```python
from build123d import *

# Parameters (mm, degrees)
SKETCH1_R               = 16
BOSS_EXTRUDE1_DEPTH     = 146
SKETCH2_W               = 150.836885197
SKETCH2_H               = 19.135619971
CUT_EXTRUDE2_DEPTH      = 17
CUT_EXTRUDE2_DEPTH_BACK = 17
SKETCH3_R               = 4
CUT_EXTRUDE3_DEPTH      = 15.463502114
CUT_EXTRUDE3_DEPTH_BACK = 15.463502114
SKETCH5_W               = 20
SKETCH5_H               = 24.196648242
CUT_EXTRUDE4_DEPTH      = 17.0000001
CUT_EXTRUDE4_DEPTH_BACK = 17.0000001
SKETCH6_R               = 4
CUT_EXTRUDE5_DEPTH      = 29


with BuildPart() as part:
    # Sketch1 → Boss-Extrude1 (new body)
    with BuildSketch(Plane.XY):
        Circle(SKETCH1_R)
    extrude(amount=BOSS_EXTRUDE1_DEPTH)

    # Sketch2 → Cut-Extrude2 (cut, two sides)
    with BuildSketch(Plane(origin=(0, 0, 0), x_dir=(0, 0, -1), z_dir=(1, 0, 0))) as cut_extrude2_sk:
        with BuildLine():
            Line((-116, -5), (-116, 5))
            ThreePointArc((-116, 5), (-116.878679656, 7.121320344), (-119, 8))
            Line((-119, 8), (-146, 8))
            Line((-146, 8), (-146, -8))
            Line((-146, -8), (-119, -8))
            ThreePointArc((-119, -8), (-116.878679656, -7.121320344), (-116, -5))
        make_face()
        with Locations((-70.581557402, -24.031312)):
            Rectangle(SKETCH2_W, SKETCH2_H)
        with Locations((-70.581557402, 24.031312)):
            Rectangle(SKETCH2_W, SKETCH2_H)
    extrude(amount=CUT_EXTRUDE2_DEPTH, mode=Mode.SUBTRACT)
    extrude(cut_extrude2_sk.sketch, amount=-CUT_EXTRUDE2_DEPTH_BACK, mode=Mode.SUBTRACT)

    # Sketch3 → Cut-Extrude3 (cut, two sides)
    with BuildSketch(Plane(origin=(0, 0, 0), x_dir=(1, 0, 0), z_dir=(0, 1, 0))) as cut_extrude3_sk:
        with Locations((0, -136)):
            Circle(SKETCH3_R)
    extrude(amount=CUT_EXTRUDE3_DEPTH, mode=Mode.SUBTRACT)
    extrude(cut_extrude3_sk.sketch, amount=-CUT_EXTRUDE3_DEPTH_BACK, mode=Mode.SUBTRACT)

    # Sketch4 → Cut-Revolve3 (revolve, cut)
    with BuildSketch(Plane(origin=(0, 0, 0), x_dir=(0, 0, -1), z_dir=(1, 0, 0))):
        with BuildLine():
            Line((0, 7), (-80, 7))
            ThreePointArc((-80, 7), (-86.772424654, 8.019684618), (-92.944350416, 10.988324842))
            Line((-92.944350416, 10.988324842), (-118.219798108, 28.197447612))
            Line((-118.219798108, 28.197447612), (0, 28.197447612))
            Line((0, 28.197447612), (0, 7))
        make_face()
    revolve(axis=Axis((0, 0, 0), (0, 0, 1)), mode=Mode.SUBTRACT)

    # Sketch5 → Cut-Extrude4 (cut, two sides)
    with BuildSketch(Plane(origin=(0, 0, 0), x_dir=(0, 0, -1), z_dir=(1, 0, 0))) as cut_extrude4_sk:
        with Locations((-10, 0)):
            Rectangle(SKETCH5_W, SKETCH5_H)
    extrude(amount=CUT_EXTRUDE4_DEPTH, mode=Mode.SUBTRACT)
    extrude(cut_extrude4_sk.sketch, amount=-CUT_EXTRUDE4_DEPTH_BACK, mode=Mode.SUBTRACT)

    # Sketch6 → Cut-Extrude5 (cut)
    with BuildSketch(Plane(origin=(0, 0, 20), x_dir=(-1, 0, 0), z_dir=(0, 0, -1))):
        Circle(SKETCH6_R)
    extrude(amount=-CUT_EXTRUDE5_DEPTH, mode=Mode.SUBTRACT)


solid = part.part
```
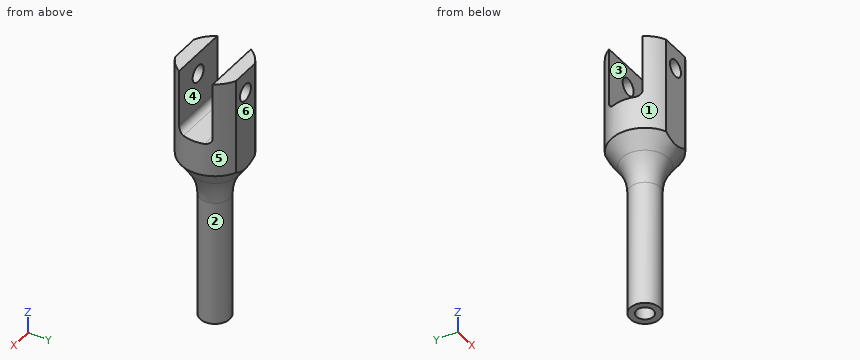
Here's how the part is built. I have some questions about the finished solid (model axes, mm). Face numbers are marked on the shaded views. A direction names the side the tool comes from. Give positions to 0.01 mm unless a question says otherwise; leave off trailing zeros. Loops run counter-clockwise (first coordinate to the right, second up) from the corner with the lowest first, then second, coordinate; pieces in that order, holes last. Notation, with made-up numbers: M -25,-27.5 L 15,-27.5 A33 ccw 15,4.5 Z; hole C 83.25,34.5 d9. An arc over 180 degrees is marked long. Put each result on its own line as item: value. Start each with the question number.
(1) Will these pins go through, and if not, where does the flat tip stop? pin 1 Ø8 at (x, z) = (-1, 33) entering from +Y; pin 2 Ø7 at (x, y) = (0, 0) entering from +Z; pin 3 Ø6 at (x, y) = (3, 4.5) entering from +Z.
(2) I need wall thicknesses on line 1 along Y through (x, z) = (0, 39); line 2 along Z through (x, y) = (0, -12); line 3 along X through (y, z) = (-9.5, 136). Which ranges of each line are inside material? Lowest first, please. Write a range as [from, to].
(3) If we mould it in two halves opening along Y, with no side actions, what happens to the marked faces 4, 5 and 6? For each: +Y half, -Y half, draft (parallel to the pull), parting line (faces both ways), or undercut.
(4) I want a section at C-C on z = 136. Please give me the cut outline in (x, y).
(5) I want a section at A-A on x = 0. Please give me the cut outline in (y, z), then the cut area to 3 significant figures.
(6) I want a section at B-B on y = 0. Please give me the cut outline in (x, z).
(7) For the marked faces 1, 2 and 3, which set-ups out of +Z, -Z, +X, -X, +Y, -Y let a thin tool reach every point of the face, with its end or its side?
(8) I want a section at D-D on z = 54. Please give me the cut outline in (x, y), then the cut area to 3 significant figures.
Answer block:
1. pin 1: y = 7
1. pin 2: z = 116
1. pin 3: z = 117.34
2. line 1: [-7, -4], [4, 7]
2. line 2: [94.43, 132], [140, 146]
2. line 3: [-12.87, -4], [4, 12.87]
3. face 4: undercut
3. face 5: parting line
3. face 6: +Y half
4. outline: M -13.86,-8 A16 ccw -6.84,-14.46 L -4,-14.46 L -4,-8 Z; M -13.86,8 L -4,8 L -4,14.46 L -6.84,14.46 A16 ccw Z; M 4,-14.46 L 6.84,-14.46 A16 ccw 13.86,-8 L 4,-8 Z; M 4,8 L 13.86,8 A16 ccw 6.84,14.46 L 4,14.46 Z
5. outline: M -14.46,98.05 L -10.99,92.94 A23 cw -7,80 L -7,20 L -4,20 L -4,49 L 4,49 L 4,20 L 7,20 L 7,80 A23 cw 10.99,92.94 L 14.46,98.05 L 14.46,132 L 8,132 L 8,119 A3 cw 5,116 L -5,116 A3 cw -8,119 L -8,132 L -14.46,132 Z; M -14.46,140 L -8,140 L -8,146 L -14.46,146 Z; M 8,140 L 14.46,140 L 14.46,146 L 8,146 Z
5. area: 1,760 mm^2
6. outline: M -16,100.31 L -10.99,92.94 A23 cw -7,80 L -7,20 L -4,20 L -4,49 L 4,49 L 4,20 L 7,20 L 7,80 A23 cw 10.99,92.94 L 16,100.31 L 16,116 L -16,116 Z
7. face 1: +Z, -Z, -X
7. face 2: -Z
7. face 3: +Z, +X, -X
8. outline: C 0,0 d14
8. area: 154 mm^2
